```python
from build123d import *

# Parameters (mm, degrees)
SKETCH_1_W          = 93.4
SKETCH_1_H          = 55.6
SKETCH_1_R          = 1.6
EXTRUDE_1_DEPTH     = 2
CUT_EXTRUDE_1_DEPTH = 60.182598794
FILLET_1_R          = 3


with BuildPart() as part:
    # 草图1 → 凸台-拉伸1 (new body)
    with BuildSketch(Plane.XY):
        with Locations((0, -8.5)):
            Rectangle(SKETCH_1_W, SKETCH_1_H)
        with Locations((-40, -26.3)):
            Circle(SKETCH_1_R, mode=Mode.SUBTRACT)
        with Locations((40, -26.3)):
            Circle(SKETCH_1_R, mode=Mode.SUBTRACT)
        with BuildLine():
            ThreePointArc((-42.7, 10.41328679), (-43.95930804, 12.856643395), (-42.7, 15.3))
            ThreePointArc((-42.7, 15.3), (-40.95930804, 15.856643395), (-39.218616079, 15.3))
            Line((-39.218616079, 15.3), (-24.381383921, 15.3))
            ThreePointArc((-24.381383921, 15.3), (-22.64069196, 15.856643395), (-20.9, 15.3))
            ThreePointArc((-20.9, 15.3), (-19.974039013, 14.231038556), (-19.64069196, 12.856643395))
            ThreePointArc((-19.64069196, 12.856643395), (-19.974039013, 11.482248234), (-20.9, 10.41328679))
            Line((-20.9, 10.41328679), (-20.9, -10.41328679))
            ThreePointArc((-20.9, -10.41328679), (-19.974039013, -11.482248234), (-19.64069196, -12.856643395))
            ThreePointArc((-19.64069196, -12.856643395), (-19.974039013, -14.231038556), (-20.9, -15.3))
            ThreePointArc((-20.9, -15.3), (-22.64069196, -15.856643395), (-24.381383921, -15.3))
            Line((-24.381383921, -15.3), (-39.218616079, -15.3))
            ThreePointArc((-39.218616079, -15.3), (-40.95930804, -15.856643395), (-42.7, -15.3))
            ThreePointArc((-42.7, -15.3), (-43.95930804, -12.856643395), (-42.7, -10.41328679))
            Line((-42.7, -10.41328679), (-42.7, 10.41328679))
        make_face(mode=Mode.SUBTRACT)
        with BuildLine():
            ThreePointArc((-10.9, 10.41328679), (-12.15930804, 12.856643395), (-10.9, 15.3))
            ThreePointArc((-10.9, 15.3), (-9.15930804, 15.856643395), (-7.418616079, 15.3))
            Line((-7.418616079, 15.3), (7.418616079, 15.3))
            ThreePointArc((7.418616079, 15.3), (9.15930804, 15.856643395), (10.9, 15.3))
            ThreePointArc((10.9, 15.3), (11.825960987, 14.231038556), (12.15930804, 12.856643395))
            ThreePointArc((12.15930804, 12.856643395), (11.825960987, 11.482248234), (10.9, 10.41328679))
            Line((10.9, 10.41328679), (10.9, -10.41328679))
            ThreePointArc((10.9, -10.41328679), (11.825960987, -11.482248234), (12.15930804, -12.856643395))
            ThreePointArc((12.15930804, -12.856643395), (11.825960987, -14.231038556), (10.9, -15.3))
            ThreePointArc((10.9, -15.3), (9.15930804, -15.856643395), (7.418616079, -15.3))
            Line((7.418616079, -15.3), (-7.418616079, -15.3))
            ThreePointArc((-7.418616079, -15.3), (-9.15930804, -15.856643395), (-10.9, -15.3))
            ThreePointArc((-10.9, -15.3), (-12.15930804, -12.856643395), (-10.9, -10.41328679))
            Line((-10.9, -10.41328679), (-10.9, 10.41328679))
        make_face(mode=Mode.SUBTRACT)
        with BuildLine():
            ThreePointArc((20.9, 10.41328679), (19.64069196, 12.856643395), (20.9, 15.3))
            ThreePointArc((20.9, 15.3), (22.64069196, 15.856643395), (24.381383921, 15.3))
            Line((24.381383921, 15.3), (39.218616079, 15.3))
            ThreePointArc((39.218616079, 15.3), (40.95930804, 15.856643395), (42.7, 15.3))
            ThreePointArc((42.7, 15.3), (43.625960987, 14.231038556), (43.95930804, 12.856643395))
            ThreePointArc((43.95930804, 12.856643395), (43.625960987, 11.482248234), (42.7, 10.41328679))
            Line((42.7, 10.41328679), (42.7, -10.41328679))
            ThreePointArc((42.7, -10.41328679), (43.625960987, -11.482248234), (43.95930804, -12.856643395))
            ThreePointArc((43.95930804, -12.856643395), (43.625960987, -14.231038556), (42.7, -15.3))
            ThreePointArc((42.7, -15.3), (40.95930804, -15.856643395), (39.218616079, -15.3))
            Line((39.218616079, -15.3), (24.381383921, -15.3))
            ThreePointArc((24.381383921, -15.3), (22.64069196, -15.856643395), (20.9, -15.3))
            ThreePointArc((20.9, -15.3), (19.64069196, -12.856643395), (20.9, -10.41328679))
            Line((20.9, -10.41328679), (20.9, 10.41328679))
        make_face(mode=Mode.SUBTRACT)
    extrude(amount=EXTRUDE_1_DEPTH)

    # 草图2 → 切除-拉伸1 (cut, through all)
    with BuildSketch(Plane.XY.offset(2)):
        with BuildLine():
            Line((-28, -31.3), (-28, -21.3))
            ThreePointArc((-28, -21.3), (-27, -20.3), (-26, -21.3))
            Line((-26, -21.3), (-26, -25.3))
            Line((-26, -25.3), (-22, -25.3))
            Line((-22, -25.3), (-22, -21.3))
            ThreePointArc((-22, -21.3), (-21, -20.3), (-20, -21.3))
            Line((-20, -21.3), (-20, -31.3))
            ThreePointArc((-20, -31.3), (-21, -32.3), (-22, -31.3))
            Line((-22, -31.3), (-22, -27.3))
            Line((-22, -27.3), (-26, -27.3))
            Line((-26, -27.3), (-26, -31.3))
            ThreePointArc((-26, -31.3), (-27, -32.3), (-28, -31.3))
        make_face()
        with BuildLine():
            Line((-12, -21.3), (-12, -28.3))
            ThreePointArc((-12, -28.3), (-8, -32.3), (-4, -28.3))
            Line((-4, -28.3), (-4, -21.3))
            ThreePointArc((-4, -21.3), (-5.05, -20.25), (-6.1, -21.3))
            Line((-6.1, -21.3), (-6.1, -28.3))
            ThreePointArc((-6.1, -28.3), (-8, -30.2), (-9.9, -28.3))
            Line((-9.9, -28.3), (-9.9, -21.3))
            ThreePointArc((-9.9, -21.3), (-10.95, -20.25), (-12, -21.3))
        make_face()
        with BuildLine():
            Line((19, -22.3), (22, -22.3))
            Line((22, -22.3), (22, -31.3))
            ThreePointArc((22, -31.3), (23, -32.3), (24, -31.3))
            Line((24, -31.3), (24, -22.3))
            Line((24, -22.3), (27, -22.3))
            ThreePointArc((27, -22.3), (28, -21.3), (27, -20.3))
            Line((27, -20.3), (19, -20.3))
            ThreePointArc((19, -20.3), (18, -21.3), (19, -22.3))
        make_face()
        with BuildLine():
            ThreePointArc((8, -25.3), (10.776736691, -30.930665002), (4.619259608, -29.705866658))
            ThreePointArc((4.619259608, -29.705866658), (5.326366389, -28.481121786), (6.551111261, -29.188228568))
            ThreePointArc((6.551111261, -29.188228568), (9.19003001, -29.713142144), (8, -27.3))
            ThreePointArc((8, -27.3), (5.223263309, -21.669334998), (11.380740392, -22.894133342))
            ThreePointArc((11.380740392, -22.894133342), (10.673633611, -24.118878214), (9.448888739, -23.411771432))
            ThreePointArc((9.448888739, -23.411771432), (6.80996999, -22.886857856), (8, -25.3))
        make_face()
    extrude(amount=-CUT_EXTRUDE_1_DEPTH, mode=Mode.SUBTRACT)

    # 圆角1
    fillet_1_edges = [part.edges().sort_by_distance(p)[0] for p in [
        (-46.7, -36.3, 1),
        (-46.7, 19.3, 1),
        (46.7, 19.3, 1),
        (46.7, -36.3, 1),
    ]]
    fillet(fillet_1_edges, radius=FILLET_1_R)


solid = part.part
```
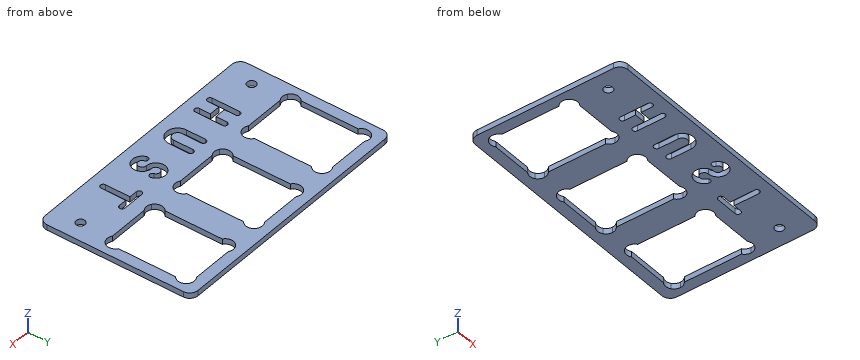
Source: CAD feature listing. Evaluate the final solid. Frame: model axes, mm. Coordinates: 2 decimals unless noted, no trailing zeros. Order: outer loops, then holes, each group sorted by start corner. A loop starts at its lowest first (then second) coordinate and runs counter-clockwise, first axis right, second up. Notation, with made-up numbers: M 64,4 L 121,4 A35 ccw 121,37 Z; hole C 17.25,-30 d6. An arc over 180 degrees is marked long. Write each question's results on one line, items separated by ' | '. Start each with the question number.
1) Section query C-C (x = 25.5). Return the cut outline in (y, z).
2) Line query: line 1 (X direction, y = -9.5, z = 1.2); line 2 (Y direction, x = -25, z = 0.25); line 3 (Y direction, x = 2, z = 1.75). Output: solid intervals per line, ascending. Write a range as from..to.
3) Section query D-D (z = 1.3). Give the number of separate pieces and of enclosed holes in the cut face, plus the area to 3 significant figures.
4) Section query B-B (x = 2). Return the cut outline in (y, z), plus the area to 3 significant figures.
5) Section query A-A (y = 7). Return the cut outline in (x, z), plus the area to 3 significant figures.
Answers:
1) outline: M -36.3,0 L -22.3,0 L -22.3,2 L -36.3,2 Z; M -20.3,0 L -15.3,0 L -15.3,2 L -20.3,2 Z; M 15.3,0 L 19.3,0 L 19.3,2 L 15.3,2 Z
2) line 1: x = -46.7..-42.7, -20.9..-10.9, 10.9..20.9, 42.7..46.7 | line 2: y = -36.3..-27.3, -25.3..-15.3, 15.3..19.3 | line 3: y = -36.3..-15.3, 15.3..19.3
3) separate pieces: 1 | enclosed holes: 9 | area: 2,910 mm^2
4) outline: M -36.3,0 L -15.3,0 L -15.3,2 L -36.3,2 Z; M 15.3,0 L 19.3,0 L 19.3,2 L 15.3,2 Z | area: 50.0 mm^2
5) outline: M -46.7,0 L -42.7,0 L -42.7,2 L -46.7,2 Z; M -20.9,0 L -10.9,0 L -10.9,2 L -20.9,2 Z; M 10.9,0 L 20.9,0 L 20.9,2 L 10.9,2 Z; M 42.7,0 L 46.7,0 L 46.7,2 L 42.7,2 Z | area: 56.0 mm^2
